Solid Edge part; units mm, degrees
sketch "Sketch1" plane through (0, 0, 0) normal (0, 0, 1) x (1, 0, 0)
  circle A0 centre (-120, 0) radius 5
  circle A1 centre (84.8528, 84.8528) radius 5
  circle A2 centre (-84.8528, -84.8528) radius 5
  circle A3 centre (0, -120) radius 5
  circle A4 centre (84.8528, -84.8528) radius 5
  circle A5 centre (120, 0) radius 5
  circle A6 centre (0, 120) radius 5
  circle A7 centre (-84.8528, 84.8528) radius 5
  circle A8 centre (0, 0) radius 150
extrude "Protrusion1" add sketch "Sketch1" along normal blind 12.7
sketch "Sketch2" plane through (0, 0, 12.7) normal (0, 0, 1) x (1, 0, 0)
  arc A0 (-90.0741, -65.0445) -> (-90.0741, 65.0445) centre (0, 0) ccw
  arc A1 (-90.0741, 65.0445) -> (-90.0741, -65.0445) centre (-184.9119, 0) cw
extrude "ProtrusiónExtruida_2" add sketch "Sketch2" along normal blind 10
sketch "Sketch3" plane through (-109.956, 0, 12.7) normal (0, 0, 1) x (1, 0, 0)
  circle A0 centre (-10.044, 0) radius 7.5
extrude "ProtrusiónExtruida_3" add sketch "Sketch3" along normal blind 2
sketch "Sketch4" plane through (-120, 0, 14.7) normal (0, 0, 1) x (1, 0, 0)
  circle A0 centre (0, 0) radius 5
extrude "ProtrusiónExtruida_4" add sketch "Sketch4" along normal blind 50
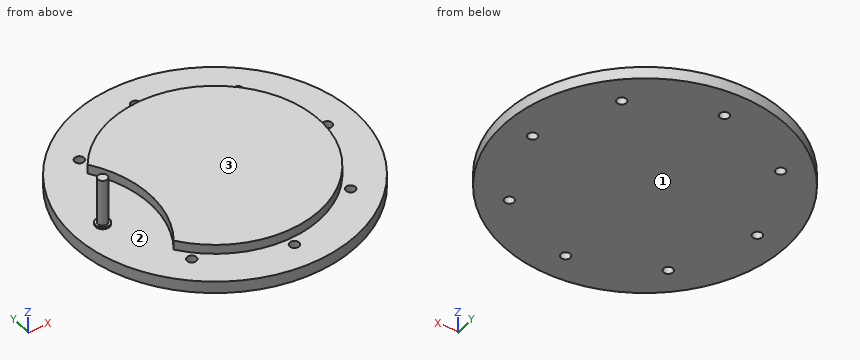
Check sheet for the modelled part. Datum: model origin and axes. Units: mm. Face numbers are marked on the shaded views. A direction names the side the tool comes from. Coordinates: 2 decimals unless noted, no trailing zeros. Order: outer loops, then holes, each group sorted by start corner. A loop starts at its lowest first (then second) coordinate and runs counter-clockwise, first axis right, second up. Notation, with made-up numbers: (-23, 60) -> (21, 60) arc R27 ccw to (21, 96) -> close; hole circle Ø6 at (-23.75, 72.5). An arc over 180 degrees is marked (long way). Write each question's results on one line, items separated by ' | '. Start each with the question number.
1) Section check A-A (x = 0). Enter the section's corners in (y, z).
2) Depth check by flat-ended pin: pin 1 (8 mm diameter, centred on x = 120, y = 0, fed in from -Z); pin 2 (1 mm diameter, centred on x = -30.5, y = -25, fed in from +Z); pin 3 (13 mm diameter, centred on x = 0, y = -120, fed in from +Z); pin 4 (12 mm diameter, centred on y = 12.5, z = 22.5, fed in from +X). Enter the tip coordinate at first touch or a pass-through.
3) Section check B-B (y = 0). Enter the section's corners in (x, z), and give its area (3 significant figures).
4) Material ranges on line 1 along Y through (x, z) = (0, 4); line 2 along Y through (x, z) = (84, 3); line 3 along Z through (x, y) = (9, -92), recorded low to high.
5) Section check C-C (x = 120). Enter the section's corners in (y, z), and give its area (3 significant figures).
6) Section check D-D (x = -120). Enter the section's corners in (y, z), and give its area (3 significant figures).
7) Set-up check for the marked faces 1, 2 and 3: record each of +Z, -Z, +X, -X, +Y, -Y from which the full face is reachable in a straight line by a thin tool's end or side.
Checked values:
1) outline: (-150, 0) -> (-125, 0) -> (-125, 12.7) -> (-150, 12.7) -> close; (-115, 0) -> (115, 0) -> (115, 12.7) -> (111.1, 12.7) -> (111.1, 22.7) -> (-111.1, 22.7) -> (-111.1, 12.7) -> (-115, 12.7) -> close; (125, 0) -> (150, 0) -> (150, 12.7) -> (125, 12.7) -> close
2) pin 1: through | pin 2: z = 22.7 | pin 3: z = 12.7 | pin 4: x = 110.91
3) outline: (-150, 0) -> (-125, 0) -> (-125, 12.7) -> (-115, 12.7) -> (-115, 0) -> (115, 0) -> (115, 12.7) -> (111.1, 12.7) -> (111.1, 22.7) -> (-69.91, 22.7) -> (-69.91, 12.7) -> (-112.5, 12.7) -> (-112.5, 14.7) -> (-115, 14.7) -> (-115, 64.7) -> (-125, 64.7) -> (-125, 14.7) -> (-127.5, 14.7) -> (-127.5, 12.7) -> (-150, 12.7) -> close; (125, 0) -> (150, 0) -> (150, 12.7) -> (125, 12.7) -> close | area: 5,900 mm²
4) line 1: -150 to -125, -115 to 115, 125 to 150 | line 2: -124.27 to -89.78, -79.93 to 79.93, 89.78 to 124.27 | line 3: 0 to 22.7
5) outline: (-90, 0) -> (-5, 0) -> (-5, 12.7) -> (-90, 12.7) -> close; (5, 0) -> (90, 0) -> (90, 12.7) -> (5, 12.7) -> close | area: 2,160 mm²
6) outline: (-90, 0) -> (-5, 0) -> (-5, 12.7) -> (5, 12.7) -> (5, 0) -> (90, 0) -> (90, 12.7) -> (7.5, 12.7) -> (7.5, 14.7) -> (5, 14.7) -> (5, 64.7) -> (-5, 64.7) -> (-5, 14.7) -> (-7.5, 14.7) -> (-7.5, 12.7) -> (-90, 12.7) -> close | area: 2,690 mm²
7) face 1: -Z, +X, -X, +Y, -Y | face 2: +Z | face 3: +Z, +X, +Y, -Y
